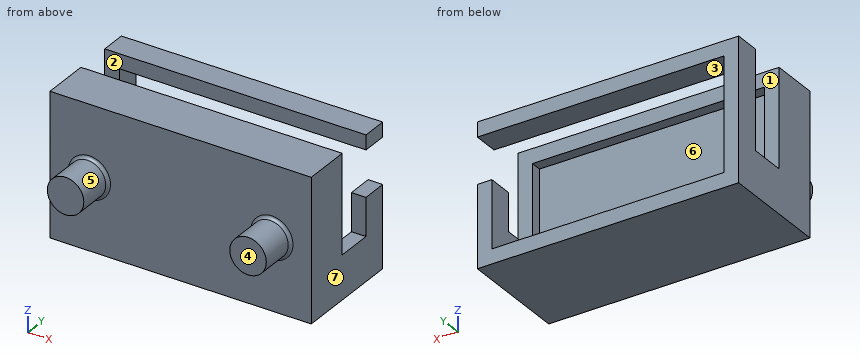
from build123d import *

# Parameters (mm, degrees)
SKETCH1_W           = 35.8
SKETCH1_H           = 19.5
SKETCH1_W_2         = 31.8
SKETCH1_H_2         = 15.5
BOSS_EXTRUDE1_DEPTH = 10
SKETCH1_2_W         = 35.8
SKETCH1_2_H         = 19.5
SKETCH1_2_W_2       = 31.8
SKETCH1_2_H_2       = 15.5
BOSS_EXTRUDE2_DEPTH = 5
SKETCH2_W           = 35.8
SKETCH2_H           = 5
CUT_EXTRUDE1_DEPTH  = 13.5
SKETCH3_W           = 6.3
SKETCH3_H           = 3.5
CUT_EXTRUDE2_DEPTH  = 2
SKETCH4_R           = 2.5
BOSS_EXTRUDE3_DEPTH = 5
FILLET1_R           = 0.4


with BuildPart() as part:
    # Sketch1 → Boss-Extrude1 (new body)
    with BuildSketch(Plane(origin=(0, 0, 0), x_dir=(1, 0, 0), z_dir=(0, 1, 0))):
        with Locations((15.9, 7.75)):
            Rectangle(SKETCH1_W, SKETCH1_H)
        with Locations((15.9, 7.75)):
            Rectangle(SKETCH1_W_2, SKETCH1_H_2, mode=Mode.SUBTRACT)
    extrude(amount=BOSS_EXTRUDE1_DEPTH)

    # Sketch1<2> → Boss-Extrude2 (add)
    # profile 1 of 2: a face of its own
    with BuildSketch(Plane(origin=(0, 0, 0), x_dir=(1, 0, 0), z_dir=(0, 1, 0))):
        with Locations((15.9, 7.75)):
            Rectangle(SKETCH1_2_W, SKETCH1_2_H)
        with Locations((15.9, 7.75)):
            Rectangle(SKETCH1_2_W_2, SKETCH1_2_H_2, mode=Mode.SUBTRACT)
    # profile 2 of 2: a face of its own
    with BuildSketch(Plane(origin=(0, 0, 0), x_dir=(1, 0, 0), z_dir=(0, 1, 0))):
        with Locations((15.9, 7.75)):
            Rectangle(SKETCH1_2_W_2, SKETCH1_2_H_2)
    extrude(amount=-BOSS_EXTRUDE2_DEPTH)

    # Sketch2 → Cut-Extrude1 (cut)
    with BuildSketch(Plane.XY.offset(2)):
        with Locations((15.9, 4)):
            Rectangle(SKETCH2_W, SKETCH2_H)
    extrude(amount=-CUT_EXTRUDE1_DEPTH, mode=Mode.SUBTRACT)

    # Sketch3 → Cut-Extrude2 (cut)
    with BuildSketch(Plane(origin=(33.8, 0, 0), x_dir=(0, 0, -1), z_dir=(1, 0, 0))):
        with Locations((3.15, 8.25)):
            Rectangle(SKETCH3_W, SKETCH3_H)
    extrude(amount=-CUT_EXTRUDE2_DEPTH, mode=Mode.SUBTRACT)

    # Sketch4 → Boss-Extrude3 (add)
    with BuildSketch(Plane.XZ.offset(5)):
        with Locations(Location((3.4, -7.75, 0), (0, 0, 90))):
            Circle(SKETCH4_R)
        with Locations(Location((28.4, -7.75, 0), (0, 0, 90))):
            Circle(SKETCH4_R)
    extrude(amount=BOSS_EXTRUDE3_DEPTH)

    # Fillet1
    fillet1_edges = [part.edges().sort_by_distance(p)[0] for p in [
        (3.4, -5, -10.25),
        (28.4, -5, -10.25),
    ]]
    fillet(fillet1_edges, radius=FILLET1_R)


solid = part.part
Can you work these out from the model? Positions are in its coordinate system, mm. Face numbers are marked on the shaded views. A direction names the side the tool comes from. Give positions to 0.01 mm unless a question says otherwise; leave off trailing zeros. Order: outer loops, then holes, each group sorted by start corner. A loop starts at its lowest first (then second) coordinate and runs counter-clockwise, first axis right, second up. Notation, with made-up numbers: M 48.5,-33 L 99.5,-33 A32 ccw 99.5,-4 Z; hole C 29.5,14 d9. An arc over 180 degrees is marked long. One line per question, with ' | ' between items.
Item 1: We'd pull the mould along Y, two halves only. Please class the marked faces 1, 2, 3 and 4: released by +Y, released by -Y, zero draft, split by the parting line, or undercut.
Answer block:
face 1: undercut | face 2: undercut | face 3: zero draft | face 4: released by -Y
Item 2: Please list where these lines run through material, in increasing order: L1, parallel to X at y = 1, z = -13.5; L2, parallel to Y at x = 5, z = 1; L3, parallel to Y at x = 24.5, z = -10.5.
Answer block:
L1: x = -2 to 0, 31.8 to 33.8 | L2: y = -5 to 1.5, 6.5 to 10 | L3: y = -5 to 0
Item 3: I'm going to push flat-ended pins straight in: pin 1 Ø10 at (x, z) = (25, -9) entering from +Y; pin 2 Ø8 at (x, z) = (25.5, -14.5) entering from -Y; pin 3 Ø0.6 at (x, y) = (33, 3) entering from +Z; pin 4 Ø11 at (x, y) = (21, 3) entering from +Z. Where does each tip first touch, or does it pass through?
Answer block:
pin 1: stops at y = 0 | pin 2: stops at y = -5 | pin 3: stops at z = -11.5 | pin 4: stops at z = 2
Item 4: Suppose I cut it at C-C, the plane y = 2.5. Write out the boundary of the cut face in (x, z).
Answer block:
outline: M -2,-17.5 L 33.8,-17.5 L 33.8,-11.5 L 31.8,-11.5 L 31.8,-15.5 L 0,-15.5 L 0,-11.5 L -2,-11.5 Z
Item 5: Suppose I cut it at A-A, the plane x = 28.4. Write out the boundary of the cut face in (y, z), then the cut area to 3 significant figures.
Answer block:
outline: M -10,-10.25 L -5.4,-10.25 A0.4 cw -5,-10.65 L -5,-17.5 L 10,-17.5 L 10,-15.5 L 0,-15.5 L 0,0 L 1.5,0 L 1.5,2 L -5,2 L -5,-4.85 A0.4 cw -5.4,-5.25 L -10,-5.25 Z; M 6.5,0 L 10,0 L 10,2 L 6.5,2 Z | area: 153 mm2
Item 6: For the marked faces 5, 6 and 7, which set-ups out of +Z, -Z, +X, -X, +Y, -Y let a thin tool reach every point of the face, with its end or its side?
Answer block:
face 5: -Y | face 6: +Y | face 7: +Z, -Z, +X, +Y, -Y
Item 7: Suppose I cut it at D-D, the plane z = -12.5. Write out the boundary of the cut face in (x, y).
Answer block:
outline: M -2,-5 L 33.8,-5 L 33.8,10 L 31.8,10 L 31.8,0 L 0,0 L 0,10 L -2,10 Z
Item 8: Suppose I cut it at B-B, the plane z = -7.75. Write out the boundary of the cut face in (x, y).
Answer block:
outline: M -2,-5 L 0.5,-5 A0.4 cw 0.9,-5.4 L 0.9,-10 L 5.9,-10 L 5.9,-5.4 A0.4 cw 6.3,-5 L 25.5,-5 A0.4 cw 25.9,-5.4 L 25.9,-10 L 30.9,-10 L 30.9,-5.4 A0.4 cw 31.3,-5 L 33.8,-5 L 33.8,1.5 L 31.8,1.5 L 31.8,0 L 0,0 L 0,1.5 L -2,1.5 Z; M -2,6.5 L 0,6.5 L 0,10 L -2,10 Z; M 31.8,6.5 L 33.8,6.5 L 33.8,10 L 31.8,10 Z
